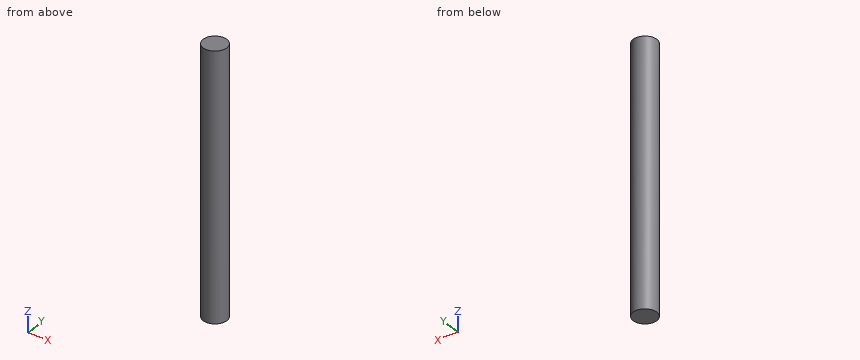
Autodesk Inventor part; units mm, degrees
ref_plane "YZ Plane" through (0, 0, 0) normal (1, 0, 0) x (0, 1, 0)
ref_plane "XZ Plane" through (0, 0, 0) normal (0, 1, 0) x (-1, 0, 0)
ref_plane "XY Plane" through (0, 0, 0) normal (0, 0, 1) x (1, 0, 0)
sketch "Szkic1" plane through (0, 0, 0) normal (0, 0, 1) x (1, 0, 0)
  circle A0 centre (-2.912, -2.7423) radius 5.3
  circle A1 centre (-2.912, -2.7423) radius 5
  point P0 (0, 0)
  dimension "d0" = 10
extrude "Wyciągnięcie proste1" add sketch "Szkic1" along normal blind 120 contours A1
move faces "Przesuń1" translate (0, 0, 5) faces at (-3.1129, -4.3968, 0)
move faces "Przesuń2" translate (0, 0, -4) faces at (-4.5787, -2.7423, 120)
properties part number "wał_2"
The listing builds one solid part. Answer for the finished solid, in the listing's coordinates (mm). Give positions to 0.01 mm unless a question says otherwise; leave off trailing zeros. Order: outer loops, then holes, each group sorted by start corner. A loop starts at its lowest first (then second) coordinate and runs counter-clockwise, first axis right, second up.
1) Find section A-A on z = 51. Write down the section's boundary in (x, y), then the cut area to 3 significant figures.
Reported:
outline: circle Ø10 at (-2.91, -2.74)
area: 78.5 mm2
2) Consider line 1 along Y through (x, z) = (1, 16); line 2 along Y through (x, z) = (-6.75, 41); line 3 along X through (y, z) = (-7, 82.5). Determine where each line is inside the solid, lowest interval first.
Reported:
line 1: y = -5.86 to 0.37
line 2: y = -5.95 to 0.46
line 3: x = -5.53 to -0.29
3) Given P1, Ø1, axis at y = -3.5, z = 68, coming from the -X side; P2, Ø1, axis at x = -6, z = 70.5, coming from the +Y side, each flat-ended and moving along its own axis, determine where each tip first touches the part or whether it passes through.
Reported:
P1: stops at x = -7.91
P2: stops at y = 1.54
4) Find section B-B on x = -6.5. Write down the section's boundary in (y, z).
Reported:
outline: (-6.22, 5) - (0.74, 5) - (0.74, 116) - (-6.22, 116) - close
5) Find section C-C on y = -6.5. Write down the section's boundary in (x, z), then the cut area to 3 significant figures.
Reported:
outline: (-6.21, 5) - (0.39, 5) - (0.39, 116) - (-6.21, 116) - close
area: 732 mm2
